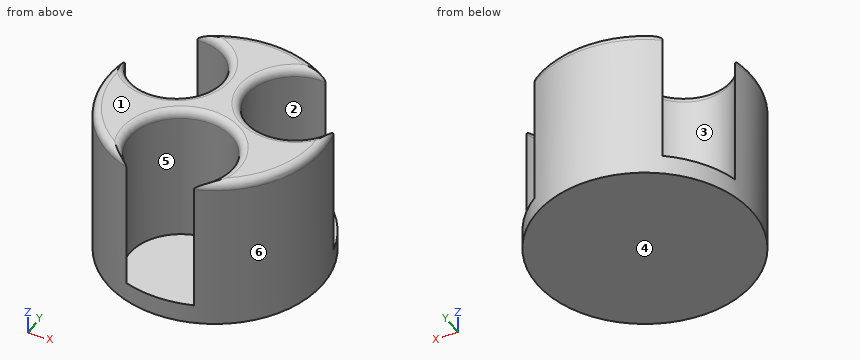
```python
from build123d import *

# Parameters (mm, degrees)
F0_R     = 27.5
F1_DEPTH = 40
F3_R     = 11.75
F3_R_2   = 12.25
F3_R_3   = 13.1
F4_DEPTH = 35
F5_R     = 2


with BuildPart() as f1:
    # F0 (on Top) → F1 (new body)
    with BuildSketch(Plane.XY):
        Circle(F0_R)
    extrude(amount=F1_DEPTH)

    # F3 (on face) → F4 (cut, through all)
    with BuildSketch(Plane.XY.offset(40)):
        with Locations((-15.416977, 10.391477)):
            Circle(F3_R)
        with Locations((15.079009, 10.054506)):
            Circle(F3_R_2)
        with Locations((0, -16.229328)):
            Circle(F3_R_3)
    extrude(amount=-F4_DEPTH, mode=Mode.SUBTRACT)

    # F5
    f5_edges = [f1.edges().sort_by_distance(p)[0] for p in [
        (22.274014, -16.128183, 40),
        (27.313425, 3.197938, 40),
        (4.886965, 3.258571, 40),
        (-0.130285, 27.499691, 40),
        (-5.673617, 3.824178, 40),
        (-24.127977, -13.194345, 40),
        (0, -3.129328, 40),
    ]]
    fillet(f5_edges, radius=F5_R)


solid = f1.part
```
Verification items for the finished model (mm, model axes). Face numbers are marked on the shaded views. A direction names the side the tool comes from. Give positions to 0.01 mm unless a question says otherwise; leave off trailing zeros. Loops run counter-clockwise (first coordinate to the right, second up) from the corner with the lowest first, then second, coordinate; pieces in that order, holes last. Notation, with made-up numbers: M 79,87.25 L 94,87.25 A25 ccw 94,114.25 Z; hole C 64,76.25 d2. An arc over 180 degrees is marked long. Return JSON: item names as keys, results as strings.
1) Material ranges on L1, parallel to Y at x = -11, z = 5.5; L2, parallel to Y at x = 11, z = 19; L3, parallel to Z at x = 12, y = 3.5, recorded low to high. Write a range as [from, to].
Findings:
{"L1": "y = [-25.2, -23.34], [-9.12, -0.5], [21.28, 25.2]", "L2": "y = [-25.2, -23.34], [-9.12, -1.5], [21.61, 25.2]", "L3": "z = [0, 5]"}
2) Tool access check on the marked faces 1 and 2. Record the directions out of +Z, -Z, +X, -X, +Y, -Y that give a thin tool (end or side, any length) a straight path to the whole face; none if there is none.
Findings:
{"face 1": "+Z, +X, -X, +Y, -Y", "face 2": "+Z"}
3) Section check C-C, the plane z = 30.5. Enter the section's corners in (x, y).
Findings:
{"outline": "M -26.63,6.87 A27.5 ccw -8.58,-26.13 A13.1 cw long 8.58,-26.13 A27.5 ccw 26.76,6.35 A12.25 cw long 16.15,22.26 A27.5 ccw -16.36,22.1 A11.75 cw long Z"}
4) Section check B-B, the plane z = 4. Enter the section's corners in (x, y).
Findings:
{"outline": "C 0,0 d55"}
5) Gauge pin test, flat ends, axial feed: P1, Ø7, axis at x = -15, y = 13, coming from the +Z side; P2, Ø2, axis at y = 12, z = 7.5, coming from the -X side; P3, Ø3, axis at x = 4, z = 32.5, coming from the +Y side. Record the tip position at first contact, or that the pin passes through.
Findings:
{"P1": "stops at z = 5", "P2": "stops at x = -3.96", "P3": "stops at y = 27.39"}
6) Mould release check, pull along Y, two halves, no side actions. Record for the marked faces 3, 4, 5 and 6: released by +Y, released by -Y, zero draft, split by the parting line, or undercut.
Findings:
{"face 3": "undercut", "face 4": "zero draft", "face 5": "undercut", "face 6": "split by the parting line"}
7) Section check A-A, the plane x = 0. Enter the section's corners in (y, z).
Findings:
{"outline": "M -27.5,0 L 27.5,0 L 27.5,38 A2 ccw 25.5,40 L -1.13,40 A2 ccw -3.13,38 L -3.13,5 L -27.5,5 Z"}
